Drawing for the job (mm, zero at the part's lowest x, y, z). A direction names the side the tool comes from. Round coordinates to 2 decimals unless told otherwise and drop trailing zeros. Write each loop counter-clockwise with the first axis right and the second up, starting at its lowest first coordinate (ties: lowest second). Pieces come first, ordered by that corner, then holes. Notation, with made-up numbers: (27.5, -2.5) -> (63.5, -2.5) arc R20 cw to (63.5, 23.5) -> close; hole circle Ø5 at (10, 28). An arc over 180 degrees is marked (long way). One line per question, with ' | ' between items.
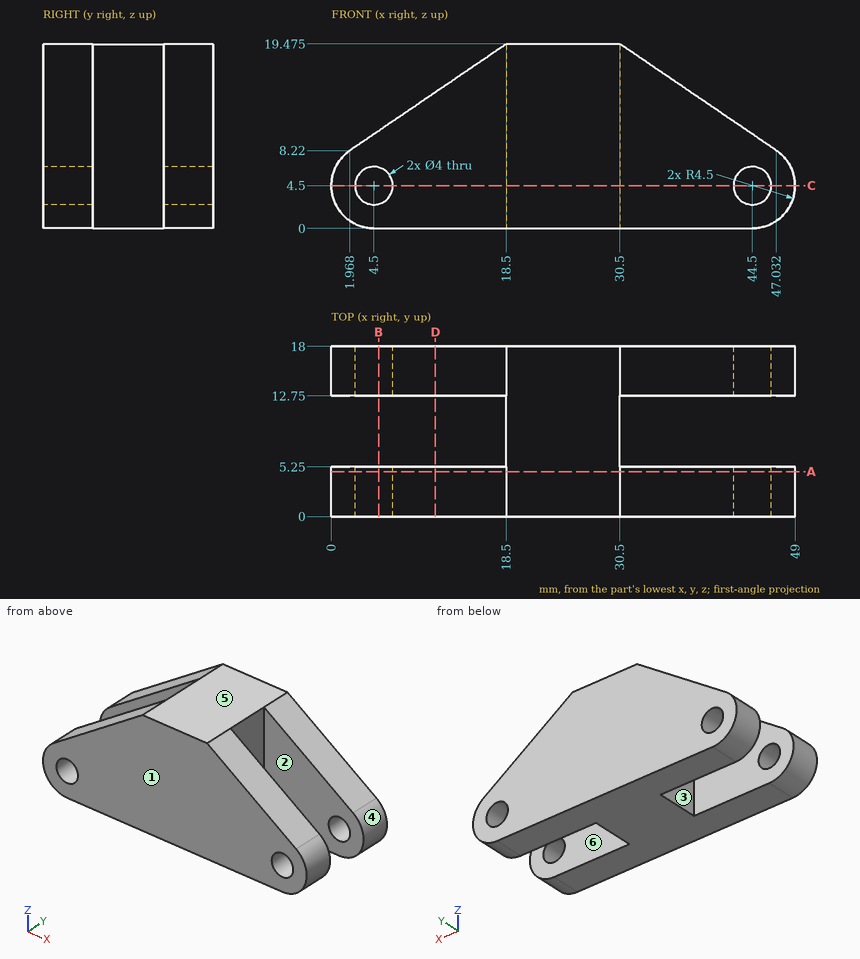
(1) Slice it at B-B (x = 5). State how many separate pieces and enclosed holes the cut face has.
Calculated:
separate pieces: 4 | enclosed holes: 0
(2) Drop flat-ended pins along their axis: pin 1 (4 mm diameter, centred on y = 6, z = 15, fed in from -X) (1 decimal); pin 2 (4 mm diameter, centred on x = 7, z = 16, fed in from +Y); pin 3 (1 mm diameter, centred on y = 5.5, z = 10, fed in from -X) (1 decimal); pin 4 (8 mm diameter, centred on y = 7.5, z = 8.5, fed in from +X). Give the stop position or say it passes through.
Calculated:
pin 1: x = 9.2 | pin 2: through | pin 3: x = 3.9 | pin 4: x = 48.95
(3) Mould opens along Y. For the marked faces 1, 2, 3 and 4 say: pulls with the +Y half, pulls with the -Y half, needs draft (parallel to the pull), parting line crosses it, or undercut.
Calculated:
face 1: pulls with the -Y half | face 2: undercut | face 3: undercut | face 4: needs draft
(4) 3-axis set-ups, long thin cutter, end or side, ignore diameter. For the marked faces 5 and 6: which of +Z, -Z, +X, -X, +Y, -Y reach the whole face in a straight line?
Calculated:
face 5: +Z, +X, -X, +Y, -Y | face 6: +Z, -Z, +X
(5) Slice it at D-D (x = 11). Write the cut outline in (y, z), then the cut area to 3 significant figures.
Calculated:
outline: (0, 0) -> (5.25, 0) -> (5.25, 14.37) -> (0, 14.37) -> close; (12.75, 0) -> (18, 0) -> (18, 14.37) -> (12.75, 14.37) -> close | area: 151 mm2
(6) Slice it at A-A (y = 4.75). Write the cut outline in (x, z) (1 decimal), then the cut area to 3 significant figures.
Calculated:
outline: (2, 8.2) arc R4.5 ccw to (4.5, 0) -> (44.5, 0) arc R4.5 ccw to (47, 8.2) -> (30.5, 19.5) -> (18.5, 19.5) -> close; hole circle Ø4 at (4.5, 4.5); hole circle Ø4 at (44.5, 4.5) | area: 686 mm2
(7) Wall check: line 1 (Y direction, x = 16.5, z = 11.25); line 2 (X direction, y = 16.25, z = 3.25) (1 decimal); line 3 (Z direction, x = 44.5, y = 3.65) (1 decimal). Give the ranges that are in metal, low to high. Write a range as from..to.
Calculated:
line 1: 0..5.25, 12.75..18 | line 2: 0.2..2.9, 6.1..42.9, 46.1..48.8 | line 3: 0..2.5, 6.5..9.9
(8) Slice it at C-C (z = 4.5). Write the cut outline in (x, y).
Calculated:
outline: (0, 0) -> (2.5, 0) -> (2.5, 5.25) -> (0, 5.25) -> close; (0, 12.75) -> (2.5, 12.75) -> (2.5, 18) -> (0, 18) -> close; (6.5, 0) -> (42.5, 0) -> (42.5, 5.25) -> (30.5, 5.25) -> (30.5, 12.75) -> (42.5, 12.75) -> (42.5, 18) -> (6.5, 18) -> (6.5, 12.75) -> (18.5, 12.75) -> (18.5, 5.25) -> (6.5, 5.25) -> close; (46.5, 0) -> (49, 0) -> (49, 5.25) -> (46.5, 5.25) -> close; (46.5, 12.75) -> (49, 12.75) -> (49, 18) -> (46.5, 18) -> close
